Build history of the part. All positions in model axes, mm. Coordinates: 2 decimals unless noted, no trailing zeros. Write each loop counter-clockwise with the first axis right and the second up, starting at its lowest first coordinate (ties: lowest second). Pieces come first, ordered by that corner, then holes.
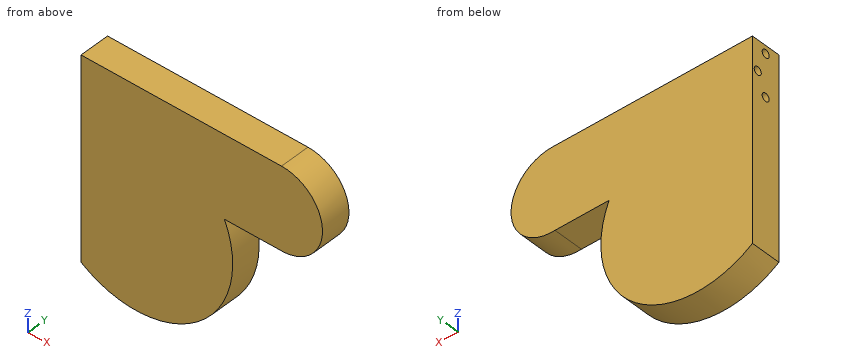
```python
from build123d import *

# Parameters (mm, degrees)
F1_DEPTH = 38.1
F3_R     = 5.08
F4_DEPTH = 63.5


with BuildPart() as f1:
    # F0 (on Front) → F1 (new body)
    with BuildSketch(Plane.XZ):
        with BuildLine():
            Line((0, 103.827015), (0, -150.172985))
            ThreePointArc((0, -150.172985), (147.702772, -143.875268), (181.698026, 0))
            Line((181.698026, 0), (250.278026, 0))
            ThreePointArc((250.278026, 0), (305.946853, 49.984613), (254, 103.827015))
            Line((254, 103.827015), (0, 103.827015))
        make_face()
    extrude(amount=F1_DEPTH)

    # F3 (on face) → F4 (cut)
    with BuildSketch(Plane(origin=(0, 0, 0), x_dir=(0, -1, 0), z_dir=(-1, 0, 0))):
        with Locations((19.05, 93.667015)):
            Circle(F3_R)
        with Locations((7.62, 65.727015)):
            Circle(F3_R)
        with Locations((19.05, 40.231943)):
            Circle(F3_R)
    extrude(amount=-F4_DEPTH, mode=Mode.SUBTRACT)


solid = f1.part
```
1. Saw through at D-D on z = -7. List the corners of the cut face in (x, y), plus the area to 3 significant figures.
Computed values:
outline: (0, -38.1) - (184.54, -38.1) - (184.54, 0) - (0, 0) - close
area: 7,030 mm2
2. Saw through at A-A on y = -7.62. List the corners of the cut face in (x, z), plus the area to 3 significant figures.
Computed values:
outline: (0, -150.17) arc R122.45 ccw to (181.7, 0) - (250.28, 0) arc R51.98 ccw (long way) to (254, 103.83) - (0, 103.83) - (0, 70.81) - (63.5, 70.81) - (63.5, 60.65) - (0, 60.65) - close
area: 59,100 mm2
3. Saw through at C-C on x = 198.5. List the corners of the cut face in (y, z).
Computed values:
outline: (-38.1, 0) - (0, 0) - (0, 103.83) - (-38.1, 103.83) - close
4. Probe line 1 along Z through (x, y) = (37, -19); line 2 along Z through (x, y) = (14, -7.62); line 3 along Z through (x, y) = (220, -23.5). List the from-to ranges inside material, lowest first.
Computed values:
line 1: z = -167.5 to 35.15, 45.31 to 88.59, 98.75 to 103.83
line 2: z = -158.54 to 60.65, 70.81 to 103.83
line 3: z = 0 to 103.83
5. Flat gauge pins, fed straight in: pin 1 (5 mm diameter, centred on y = -8.5, z = 65.5, fed in from -X); pin 2 (8 mm diameter, centred on y = -19.05, z = 40.23, fed in from +X); pin 3 (1.5 mm diameter, centred on x = 221.5, y = -5.5, fed in from -Z). Where does each tip first touch, or does it go through?
Computed values:
pin 1: stops at x = 63.5
pin 2: stops at x = 305.42
pin 3: stops at z = 0
6. Saw through at B-B on x = 19.5. List the corners of the cut face in (y, z), plus the area to 3 significant figures.
Computed values:
outline: (-38.1, -161.18) - (0, -161.18) - (0, 103.83) - (-38.1, 103.83) - close; hole circle Ø10.16 at (-19.05, 40.23); hole circle Ø10.16 at (-19.05, 93.67); hole circle Ø10.16 at (-7.62, 65.73)
area: 9,850 mm2
